Part model, mm, in its own coordinate system. A direction names the side the tool comes from. Coordinates: 2 decimals unless noted, no trailing zeros. Loops run counter-clockwise (first coordinate to the right, second up) from the corner with the lowest first, then second, coordinate; pieces in that order, holes last. Notation, with made-up numbers: M 33.25,52.5 L 44.25,52.5 A23 ccw 44.25,90.5 Z; hole C 57.5,-21.5 d5. An arc over 180 degrees is marked long. Use CSV: the item, a comma, the result in double quotes. Start each with the question number.
from build123d import *

# Parameters (mm, degrees)
SKETCH1_R           = 10.5
BOSS_EXTRUDE1_DEPTH = 1.2
SKETCH2_R           = 7.85
BOSS_EXTRUDE2_DEPTH = 11
SKETCH3_R           = 10.5
BOSS_EXTRUDE3_DEPTH = 1.2
SKETCH4_R           = 5.5
BOSS_EXTRUDE4_DEPTH = 6.6
SKETCH5_R           = 3
CUT_EXTRUDE1_DEPTH  = 21


with BuildPart() as part:
    # Sketch1 → Boss-Extrude1 (new body)
    with BuildSketch(Plane(origin=(0, 0, 0), x_dir=(1, 0, 0), z_dir=(0, 1, 0))):
        Circle(SKETCH1_R)
    extrude(amount=BOSS_EXTRUDE1_DEPTH)

    # Sketch2 → Boss-Extrude2 (add)
    with BuildSketch(Plane(origin=(0, 1.2, 0), x_dir=(1, 0, 0), z_dir=(0, 1, 0))):
        Circle(SKETCH2_R)
    extrude(amount=BOSS_EXTRUDE2_DEPTH)

    # Sketch3 → Boss-Extrude3 (add)
    with BuildSketch(Plane(origin=(0, 12.2, 0), x_dir=(1, 0, 0), z_dir=(0, 1, 0))):
        Circle(SKETCH3_R)
    extrude(amount=BOSS_EXTRUDE3_DEPTH)

    # Sketch4 → Boss-Extrude4 (add)
    with BuildSketch(Plane(origin=(0, 13.4, 0), x_dir=(1, 0, 0), z_dir=(0, 1, 0))):
        Circle(SKETCH4_R)
    extrude(amount=BOSS_EXTRUDE4_DEPTH)

    # Sketch5 → Cut-Extrude1 (cut, through all)
    with BuildSketch(Plane(origin=(0, 20, 0), x_dir=(1, 0, 0), z_dir=(0, 1, 0))):
        Circle(SKETCH5_R)
    extrude(amount=-CUT_EXTRUDE1_DEPTH, mode=Mode.SUBTRACT)


solid = part.part
1. Slice it at A-A, the plane x = 0. List the corners of the cut face in (y, z), and give its area (3 significant figures).
2. Slice it at C-C, the plane y = 16.25. List the corners of the cut face in (x, z), and give its area (3 significant figures).
3. Tool access for faces 5 (the face through (-3, 10, 0)), 6 (the face through (2, 12.2, 8)), 7 (the face through (-1.19, 16.65, 5.37)): list every direction of +Z, -Z, +X, -X, +Y, -Y with a clear straight run to the whole face (end or side of a thin tool).
4. Wall check: probe 1 along X at (y, z) = (8.25, 0); probe 2 along Y at (x, z) = (5.75, -6.75). Give the ranges that are in metal, low to high.
5. Pin check, flat tips, straight feed: pin 1 (6.5 mm diameter, centred on x = -2, z = 1, fed in from +Y); pin 2 (5 mm diameter, centred on y = 14, z = 3.5, fed in from +X) (3 decimals); pin 3 (1.5 mm diameter, centred on x = -3, y = 2, fed in from -Z); pin 4 (10 mm diameter, centred on x = -4, y = 18, fed in from +Z). Stop position of each tip, or through.
6. Slice it at B-B, the plane z = 0. List the corners of the cut face in (x, y).
7. Slice it at D-D, the plane z = 3.5. List the corners of the cut face in (x, y), and give its area (3 significant figures).
8. Two-plate mould, pull along Y, no slides. Class faces 1 (the face through (10, 0.6, -3.2)), 2 (the face through (2, 1.2, 8)), 3 (the face through (2.4, 20, 2.4)), 4 (the face through (2.2, 0, -2.5)): pulls with the +Y half, pulls with the -Y half, needs draft (parallel to the pull), parting line crosses it, or undercut.
Found:
1,outline,"M 0,-10.5 L 1.2,-10.5 L 1.2,-7.85 L 12.2,-7.85 L 12.2,-10.5 L 13.4,-10.5 L 13.4,-5.5 L 20,-5.5 L 20,-3 L 0,-3 Z; M 0,3 L 20,3 L 20,5.5 L 13.4,5.5 L 13.4,10.5 L 12.2,10.5 L 12.2,7.85 L 1.2,7.85 L 1.2,10.5 L 0,10.5 Z"
1,area,"176 mm^2"
2,outline,"C 0,0 d11; hole C 0,0 d6"
2,area,"66.8 mm^2"
3,face 5,"+Y, -Y"
3,face 6,"none"
3,face 7,"+Y"
4,probe 1,"-7.85 to -3, 3 to 7.85"
4,probe 2,"0 to 1.2, 12.2 to 13.4"
5,pin 1,"y = 20"
5,pin 2,"x = 10.445"
5,pin 3,"z = -7.52"
5,pin 4,"z = 10.3"
6,outline,"M -10.5,0 L -3,0 L -3,20 L -5.5,20 L -5.5,13.4 L -10.5,13.4 L -10.5,12.2 L -7.85,12.2 L -7.85,1.2 L -10.5,1.2 Z; M 3,0 L 10.5,0 L 10.5,1.2 L 7.85,1.2 L 7.85,12.2 L 10.5,12.2 L 10.5,13.4 L 5.5,13.4 L 5.5,20 L 3,20 Z"
7,outline,"M -9.9,0 L 9.9,0 L 9.9,1.2 L 7.03,1.2 L 7.03,12.2 L 9.9,12.2 L 9.9,13.4 L 4.24,13.4 L 4.24,20 L -4.24,20 L -4.24,13.4 L -9.9,13.4 L -9.9,12.2 L -7.03,12.2 L -7.03,1.2 L -9.9,1.2 Z"
7,area,"258 mm^2"
8,face 1,"needs draft"
8,face 2,"undercut"
8,face 3,"pulls with the +Y half"
8,face 4,"pulls with the -Y half"
